For this review, take the finished solid that the model builds, in its own axes (mm). Coordinates: 2 decimals unless noted, no trailing zeros. Loops run counter-clockwise (first coordinate to the right, second up) from the corner with the lowest first, then second, coordinate; pieces in that order, holes last.
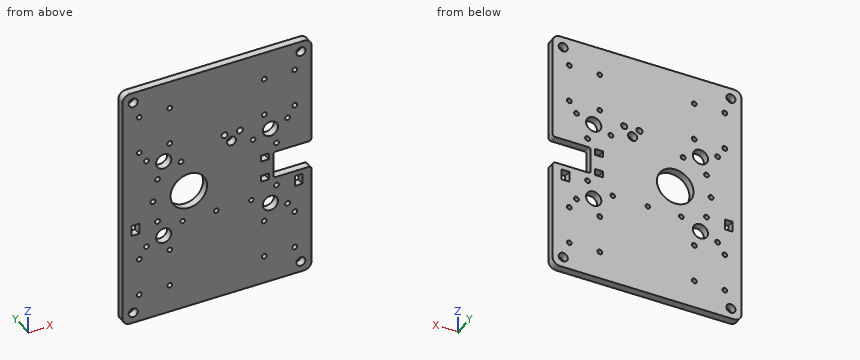
Autodesk Inventor part; units mm, degrees
ref_plane "YZ Plane" through (0, 0, 0) normal (1, 0, 0) x (0, 1, 0)
ref_plane "XZ Plane" through (0, 0, 0) normal (0, 1, 0) x (-1, 0, 0)
ref_plane "XY Plane" through (0, 0, 0) normal (0, 0, 1) x (1, 0, 0)
sketch "Sketch1" plane through (0, 0, 0) normal (0, 1, 0) x (-1, 0, 0)
  line L0 (0, 0) -> (124, 0)
  line L1 (124, 0) -> (124, -162)
  line L2 (124, -162) -> (0, -162)
  line L3 (0, -162) -> (0, 0)
  line L4 (117.9854, -81) -> (-11.1436, -81) construction
  line L5 (62, -11.2083) -> (62, -206.7638) construction
  circle A0 centre (113, -18.5) radius 1.6
  circle A1 centre (113, -43.5) radius 1.6
  circle A2 centre (93, -18.5) radius 1.6
  circle A3 centre (93, -43.5) radius 1.6
  circle A4 centre (113, -143.5) radius 1.6
  circle A5 centre (113, -118.5) radius 1.6
  circle A6 centre (93, -143.5) radius 1.6
  circle A7 centre (93, -118.5) radius 1.6
  circle A8 centre (11, -18.5) radius 1.6
  circle A9 centre (11, -43.5) radius 1.6
  circle A10 centre (31, -18.5) radius 1.6
  circle A11 centre (31, -43.5) radius 1.6
  circle A12 centre (11, -118.5) radius 1.6
  circle A13 centre (31, -143.5) radius 1.6
  circle A14 centre (11, -143.5) radius 1.6
  circle A15 centre (31, -118.5) radius 1.6
  line L6 (118, -93.5) -> (113, -93.5)
  line L7 (113, -93.5) -> (113, -100.5)
  line L8 (113, -100.5) -> (118, -100.5)
  line L9 (118, -100.5) -> (118, -93.5)
  line L10 (6, -93.5) -> (11, -93.5)
  line L11 (11, -93.5) -> (11, -100.5)
  line L12 (11, -100.5) -> (6, -100.5)
  line L13 (6, -100.5) -> (6, -93.5)
  circle A16 centre (7.5, -7.5) radius 2.8374
  circle A17 centre (37.5, -7.5) radius 2.5792
  circle A18 centre (7.5, -107.5) radius 2.9237
  circle A19 centre (37.5, -107.5) radius 2.6656
  dimension "d0" = 162
  dimension "d1" = 124
  dimension "d2" = 81
  dimension "d3" = 62
  dimension "d4" = 3.2
  dimension "d8" = 25
  dimension "d9" = 25
  dimension "d10" = 18.5
  dimension "d11" = 18.5
  dimension "d12" = 20
  dimension "d13" = 20
  dimension "d14" = 11
  dimension "d15" = 11
  dimension "d21" = 61.5
  dimension "d22" = 7
  dimension "d23" = 5
  dimension "d24" = 6
  dimension "d26" = 7.5
  dimension "d27" = 7.5
  dimension "d28" = 37.5
  dimension "d29" = 7.5
  dimension "d30" = 37.5
  dimension "d31" = 7.5
  dimension "d32" = 107.5
  dimension "d33" = 107.5
extrude "Extrusion1" add sketch "Sketch1" along normal blind 5 contours L0 L1 L2 L3 | A16 | A17 | A18 | A19
fillet "Fillet2" radius 5 4 edges at (0, 2.5, 0) (0, 2.5, -162) (-124, 2.5, -162) (-124, 2.5, 0)
sketch "Sketch3" plane through (0, 5, 0) normal (0, 1, 0) x (1, 0, 0)
  circle A0 centre (-93, 43.5) radius 1.8241
  line L0 (0, 5) -> (0, 157)
  circle A1 centre (-97, 54.8137) radius 5.6411
  circle A2 centre (-97, 54.8137) radius 16
  line L1 (-112.1751, 81) -> (15.1489, 81) construction
  line L2 (-119, 0) -> (-5, 0)
  circle A3 centre (-93, 118.5) radius 3.1
  circle A4 centre (-93, 118.5) radius 1.8241
  circle A5 centre (-97, 107.1863) radius 5.6411
  circle A6 centre (-97, 107.1863) radius 16
  circle A7 centre (-85.6863, 58.8137) radius 1.8241
  circle A8 centre (-101, 66.1274) radius 1.8241
  circle A9 centre (-108.3137, 50.8137) radius 1.8241
  circle A10 centre (-97, 54.8137) radius 5.6411
  circle A11 centre (-101, 95.8726) radius 1.8241
  circle A12 centre (-108.3137, 111.1863) radius 1.8241
  line L3 (-124, 157) -> (-124, 5)
  line L4 (-62, -8.3299) -> (-62, 205.5694) construction
  circle A13 centre (-31, 43.5) radius 3.1
  circle A14 centre (-31, 43.5) radius 1.8241
  circle A15 centre (-27, 54.8137) radius 5.6411
  circle A16 centre (-27, 54.8137) radius 16
  circle A17 centre (-31, 118.5) radius 3.1
  circle A18 centre (-31, 118.5) radius 1.8241
  circle A19 centre (-27, 107.1863) radius 5.6411
  circle A20 centre (-27, 107.1863) radius 16
  circle A21 centre (-38.3137, 58.8137) radius 1.8241
  circle A22 centre (-23, 66.1274) radius 1.8241
  circle A23 centre (-15.6863, 50.8137) radius 1.8241
  circle A24 centre (-27, 54.8137) radius 5.6411
  circle A25 centre (-15.6863, 111.1863) radius 1.8241
  circle A26 centre (-23, 95.8726) radius 1.8241
  circle A27 centre (-93, 43.5) radius 1.6
  point P0 (0, 0)
  dimension "d57" = 12
  dimension "d59" = 32
  dimension "d60" = 81
  dimension "d63" = 360
  dimension "d66" = 62
  dimension "d89" = 124
  dimension "d200" = 0
  dimension "d201" = 0
  dimension "d202" = 70
hole "Hole1" at (-108.3137, 5, -50.8137) at (-101, 5, -66.1274) at (-85.6863, 5, -58.8137) at (-108.3137, 5, -111.1863) at (-101, 5, -95.8726) at (-23, 5, -95.8726) at (-15.6863, 5, -111.1863) at (-38.3137, 5, -58.8137) at (-23, 5, -66.1274) at (-15.6863, 5, -50.8137) direction (0, -1, 0) diameter 3.2 end through all
sketch "Sketch4" plane through (0, 5, 0) normal (0, 1, 0) x (1, 0, 0)
  circle A0 centre (-97, 54.8137) radius 4
  circle A1 centre (-97, 107.1863) radius 4
  circle A2 centre (-27, 107.1863) radius 4
  circle A3 centre (-27, 54.8137) radius 4
  point P0 (0, 0)
  dimension "d203" = 70
hole "Hole2" at (-97, 5, -54.8137) at (-97, 5, -107.1863) at (-27, 5, -107.1863) at (-27, 5, -54.8137) direction (0, -1, 0) diameter 10 end through all
sketch "Sketch5" plane through (0, 5, 0) normal (0, 1, 0) x (1, 0, 0)
  circle A0 centre (-80.5, 81) radius 12
  line L0 (0, 5) -> (0, 157)
  line L1 (-119, 0) -> (-5, 0)
  circle A1 centre (-80.5, 81) radius 12 construction
  point P0 (0, 0)
  dimension "d81" = 24
  dimension "d82" = 80.5
  dimension "d83" = 81
  dimension "d90" = 24
extrude "Extrusion3" cut sketch "Sketch5" against normal blind 2
sketch "Sketch6" plane through (-80.5, 3, -81) normal (0, 1, 0) x (1, 0, 0)
  circle A0 centre (0, 0) radius 12
  point P0 (80.5, -81)
  dimension "d86" = 24
extrude "Extrusion4" cut sketch "Sketch6" against normal blind 24
sketch "Sketch7" plane through (0, 5, 0) normal (0, 1, 0) x (1, 0, 0)
  circle A0 centre (-84.5, 101) radius 1.5
  line L0 (-124, 157) -> (-124, 5)
  circle A1 centre (-62.5, 101) radius 1.5
  circle A2 centre (-39.5, 101) radius 1.5
  line L1 (-5, 162) -> (-119, 162)
  point P0 (0, 0)
  point P1 (-92.5, 103)
  point P2 (-47.5, 103)
  point P3 (-70.5, 103)
  dimension "d190" = 3
  dimension "d191" = 39.5
  dimension "d192" = 3
  dimension "d193" = 3
  dimension "d194" = 84.5
  dimension "d195" = 61.5
  dimension "d196" = 61
hole "Hole3" at (-84.5, 5, -101) at (-62.5, 5, -101) at (-39.5, 5, -101) direction (0, -1, 0) diameter 3 end through all
sketch "Sketch8" plane through (0, 5, 0) normal (0, 1, 0) x (1, 0, 0)
  line L0 (-147.8175, 81) -> (38.0677, 81) construction
  line L1 (-62, -18.8902) -> (-62, 202.7642) construction
  line L2 (-5, 162) -> (-119, 162)
  line L3 (-119, 0) -> (-5, 0)
  line L4 (0, 5) -> (0, 157)
  line L5 (-124, 157) -> (-124, 5)
  circle A0 centre (-7, 7) radius 3
  circle A1 centre (-7, 155) radius 3
  circle A2 centre (-117, 7) radius 3
  circle A3 centre (-117, 155) radius 3
  point P0 (0, 0)
  dimension "d104" = 162
  dimension "d105" = 124
  dimension "d106" = 62
  dimension "d107" = 81
  dimension "d108" = 6
  dimension "d109" = 7
  dimension "d110" = 7
hole "Hole4" at (-7, 5, -7) at (-117, 5, -7) at (-117, 5, -155) at (-7, 5, -155) direction (0, -1, 0) diameter 6 end through all
sketch "Sketch10" plane through (0, 5, 0) normal (0, 1, 0) x (1, 0, 0)
  line L0 (0, 5) -> (0, 157)
  line L1 (0, 72) -> (-25, 72)
  line L2 (-25, 72) -> (-25, 90)
  line L3 (-25, 90) -> (0, 90)
  line L4 (0, 90) -> (0, 72)
  line L5 (-119, 0) -> (-5, 0)
  line L6 (-33.2, 71.8) -> (-28, 71.8)
  line L7 (-28, 71.8) -> (-28, 76)
  line L8 (-28, 76) -> (-33.2, 76)
  line L9 (-33.2, 76) -> (-33.2, 71.8)
  line L10 (-33.2, 86) -> (-28, 86)
  line L11 (-28, 86) -> (-28, 90.2)
  line L12 (-28, 90.2) -> (-33.2, 90.2)
  line L13 (-33.2, 90.2) -> (-33.2, 86)
  point P0 (0, 0)
  point P1 (0, 90)
  dimension "d128" = 18
  dimension "d129" = 72
  dimension "d130" = 25
  dimension "d184" = 4.2
  dimension "d185" = 5.2
  dimension "d186" = 4.2
  dimension "d187" = 18.4
  dimension "d188" = 0.2
  dimension "d189" = 3
extrude "Extrusion5" cut sketch "Sketch10" against normal blind 10
fillet "Fillet4" radius 2 2 edges at (0, 2.5, -90) (0, 2.5, -72)
sketch "Sketch12" plane through (0, 0, 0) normal (0, -1, 0) x (1, 0, 0)
  circle A0 centre (-47, -49.5) radius 2
  circle A1 centre (-57, -49.5) radius 2
  line L0 (-119, 0) -> (-5, 0)
  line L1 (-40, -51) -> (-40, -46)
  circle A2 centre (-47, -49.5) radius 1.2295
  circle A3 centre (-47, -49.5) radius 1.2295
  circle A4 centre (-47, -49.5) radius 1.2295
  circle A5 centre (-57, -49.5) radius 1.2295
  point P0 (0, 0)
  dimension "d142" = 4
  dimension "d144" = 4
hole "Hole7" at (-47, 0, -49.5) at (-57, 0, -49.5) direction (0, 1, 0) diameter 4 depth 20 tip angle 118
sketch "Sketch13" plane through (0, 5, 0) normal (0, 1, 0) x (1, 0, 0)
  circle A0 centre (-104, 81) radius 1.5
  line L0 (-124, 157) -> (-124, 5)
  line L1 (-119, 0) -> (-5, 0)
  point P0 (0, 0)
  dimension "d154" = 3
  dimension "d155" = 20
  dimension "d156" = 81
hole "Hole8" at (-104, 5, -81) direction (0, -1, 0) diameter 3.2 depth 20 tip angle 118
sketch "Sketch14" plane through (0, 5, 0) normal (0, 1, 0) x (1, 0, 0)
  circle A0 centre (-52.5, 55) radius 3
  line L0 (-119, 0) -> (-5, 0)
  line L1 (0, 5) -> (0, 70)
  point P0 (0, 0)
  dimension "d164" = 55
  dimension "d165" = 52.5
  dimension "d166" = 6
hole "Hole9" at (-52.5, 5, -55) direction (0, -1, 0) diameter 6 depth 20 tip angle 118
fillet "Fillet6" radius 1.5 2 edges at (-25, 2.5, -72) (-25, 2.5, -90)
equation "\"d2\" = 0.5 * d0"
equation "\"d3\" = 0.5 * d1"
equation "\"d66\" = 0.5 * d89"
equation "\"d106\" = 0.5 * d105"
equation "\"d107\" = 0.5 * d104"
equation "\"d147\" = d144"
equation "\"d167\" = d166"
properties part number "x-Axis_plate_bottom_t" material "PET Plastic"
Q1. For pin 1 Ø4 at (x, z) = (-15.69, -50.81) entering from -Y; pin 2 Ø1.9 at (x, z) = (-11, -18.5) entering from -Y, all flat-tipped, find the tip position at first contact; note any pin that passes through.
Q2. Consider section A-A (x = -47). State the section outline as (y, z) points, then the cut area to 3 significant figures.
Q3. Wall thickness on probe 1 along X at (y, z) = (2.95, -143.5); probe 2 along Z at (x, y) = (-16, 4.1); probe 3 along Z at (x, y) = (-18, 4.3): over which ranges is each line inside the solid? List them lowest first.
Q4. Consider section B-B (x = -97). State the section outline as (y, z) points.
Q5. Consider section C-C (y = 3.1). Count the separate pieces of the cut face and the enclosed holes in it, then the cut area to 3 significant figures.
Model answer:
1. pin 1: stops at y = 0
1. pin 2: passes through
2. outline: (0, -162) - (5, -162) - (5, -51.5) - (0, -51.5) - close; (0, -47.5) - (5, -47.5) - (5, 0) - (0, 0) - close
2. area: 790 mm2
3. probe 1: x = -124 to -114.6, -111.4 to -94.6, -91.4 to -32.6, -29.4 to -12.6, -9.4 to 0
3. probe 2: z = -162 to -112.76, -109.62 to -90, -72 to -52.38, -49.24 to 0
3. probe 3: z = -162 to -90, -72 to 0
4. outline: (0, -162) - (5, -162) - (5, -112.19) - (0, -112.19) - close; (0, -102.19) - (5, -102.19) - (5, -59.81) - (0, -59.81) - close; (0, -49.81) - (5, -49.81) - (5, 0) - (0, 0) - close
5. separate pieces: 1
5. enclosed holes: 46
5. area: 18,300 mm2
